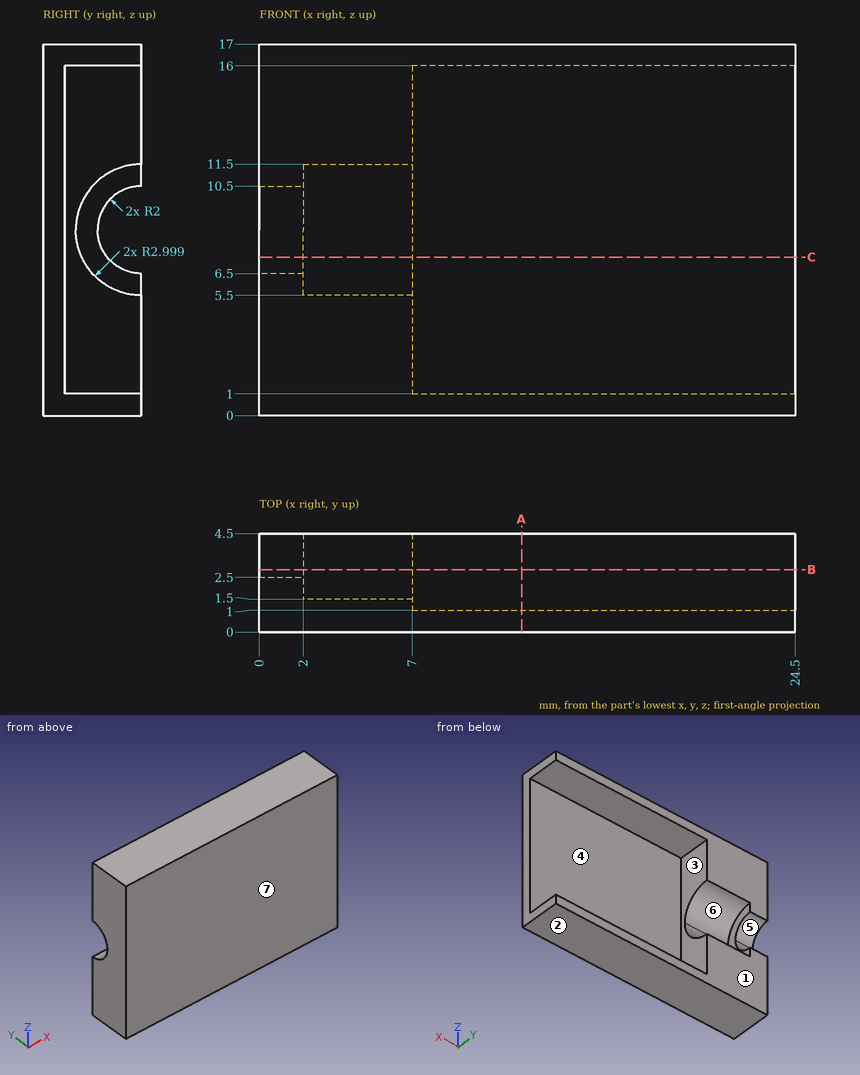
Check sheet for the drawn part. Datum: minimum x, y, z corner. Units: mm. A direction names the side the tool comes from. Round coordinates to 2 decimals unless told otherwise and drop trailing zeros. Loops run counter-clockwise (first coordinate to the right, second up) from the corner with the lowest first, then second, coordinate; pieces in that order, holes last. Notation, with made-up numbers: (3, 88) - (29, 88) arc R28 ccw to (29, 111) - close; hole circle Ø5 at (-15, 6). An arc over 180 degrees is marked (long way). Write item = value, one per line. Start each with the question number.
1. Mould release check, pull along Z, two halves, no side actions. Record for the marked faces 1, 2, 3 and 4: released by +Z, released by -Z, zero draft, split by the parting line, or undercut.
2. Depth check by flat-ended pin: pin 1 (1.5 mm diameter, centred on x = 13, z = 3.5, fed in from +Y); pin 2 (1.5 mm diameter, centred on y = 3.5, z = 8, fed in from +X). Enter the tip coordinate at first touch or a pass-through.
3. Thickness scan on line 1 (Z direction, x = 17.75, y = 1.05); line 2 (Y direction, x = 14, z = 1.5); line 3 (X direction, y = 2.35, z = 14.75). Record the ranges inside material, lowest first.
4. Section check B-B on y = 2.85. Enter the section's corners in (x, z) (1 decimal).
5. Section check A-A on x = 12. Enter the section's corners in (y, z).
6. Set-up check for the marked faces 5, 6 and 7: record each of +Z, -Z, +X, -X, +Y, -Y from which the full face is reachable in a straight line by a thin tool's end or side.
7. Section check C-C on z = 7.25. Enter the section's corners in (x, y).
Working result:
q1.face_1 = zero draft
q1.face_2 = released by -Z
q1.face_3 = undercut
q1.face_4 = undercut
q2.pin_1 = 1
q2.pin_2 = through
q3.line_1 = 0 to 1, 16 to 17
q3.line_2 = 0 to 1
q3.line_3 = 0 to 7
q4.outline = (0, 0) - (24.5, 0) - (24.5, 1) - (7, 1) - (7, 6) - (2, 6) - (2, 7.4) - (0, 7.4) - close; (0, 9.6) - (2, 9.6) - (2, 11) - (7, 11) - (7, 16) - (24.5, 16) - (24.5, 17) - (0, 17) - close
q5.outline = (0, 0) - (4.5, 0) - (4.5, 1) - (1, 1) - (1, 16) - (4.5, 16) - (4.5, 17) - (0, 17) - close
q6.face_5 = +X, -X, +Y
q6.face_6 = +X, +Y
q6.face_7 = +Z, -Z, +X, -X, -Y
q7.outline = (0, 0) - (24.5, 0) - (24.5, 1) - (7, 1) - (7, 1.77) - (2, 1.77) - (2, 2.94) - (0, 2.94) - close
